Part model, mm, in its own coordinate system. Face numbers are marked on the shaded views. Give positions to 0.01 mm unless a question says otherwise; leave off trailing zeros. Write each loop counter-clockwise with the first axis right and the second up, starting at its lowest first coordinate (ties: lowest second). Pieces come first, ordered by that corner, then holes. Notation, with made-up numbers: M 54,44 L 65,44 A16 ccw 65,74 Z; hole C -20,-4 d2. An arc over 180 degrees is marked long. Use a Markdown table: item, result.
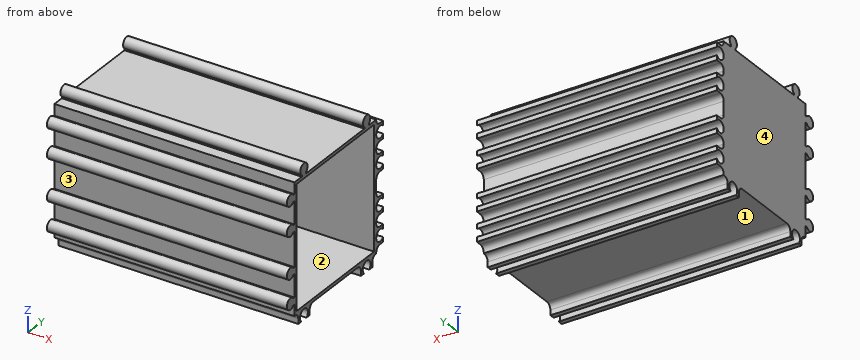
```python
from build123d import *

# Parameters (mm, degrees)
EXTRUDE_1_DEPTH             = 90
SKETCH_2_W                  = 90
SKETCH_2_H                  = 42.75
EXTRUDE_2_DEPTH             = 8.2
SKETCH_3_W                  = 90
SKETCH_3_H                  = 52.45
EXTRUDE_3_DEPTH             = 8.2
SKETCH_4_W                  = 3.95
SKETCH_4_H                  = 2.25
CUT_EXTRUDE_1_DEPTH         = 91
SKETCH_5_W                  = 3.95
SKETCH_5_H                  = 29.5
CUT_EXTRUDE_2_DEPTH         = 91
SKETCH_6_W                  = 3.95
SKETCH_6_H                  = 6.2
CUT_EXTRUDE_3_DEPTH         = 91
SKETCH_7_W                  = 2.25
SKETCH_7_H                  = 3.95
CUT_EXTRUDE_4_DEPTH         = 91
SKETCH_8_W                  = 4.5
SKETCH_8_H                  = 3.95
CUT_EXTRUDE_5_DEPTH         = 91
SKETCH_9_W                  = 9
SKETCH_9_H                  = 3.95
CUT_EXTRUDE_6_DEPTH         = 91
SKETCH_10_W                 = 4.5
SKETCH_10_H                 = 3.95
CUT_EXTRUDE_7_DEPTH         = 91
SKETCH_11_W                 = 2.25
SKETCH_11_H                 = 3.95
CUT_EXTRUDE_8_DEPTH         = 91
SKETCH_12_W                 = 46.1
SKETCH_12_H                 = 44.6
CUT_EXTRUDE_9_DEPTH         = 86.2
HOLE_WIZARD_2_5_2_5_1_D     = 2.5
HOLE_WIZARD_2_5_2_5_1_DEPTH = 90
HOLE_WIZARD_4_5_4_5_1_D     = 4.5
HOLE_WIZARD_4_5_4_5_1_DEPTH = 90
SKETCH_19_R                 = 1.67252853
SKETCH_19_R_2               = 1.459159852
SKETCH_19_R_3               = 1.459908976
SKETCH_19_R_4               = 1.592821911
SKETCH_19_R_5               = 1.532216665
SKETCH_19_R_6               = 1.596138091
EXTRUDE_4_DEPTH             = 90
FILLET_1_R                  = 2
FILLET_2_R                  = 2
FILLET_3_R                  = 2
FILLET_4_R                  = 2
FILLET_5_R                  = 2
FILLET_6_R                  = 2
FILLET_7_R                  = 2
FILLET_8_R                  = 2
FILLET_9_R                  = 2
FILLET_10_R                 = 2
FILLET_11_R                 = 2
FILLET_12_R                 = 2


with BuildPart() as part:
    # Эскиз1 → Бобышка-Вытянуть1 (new body)
    with BuildSketch(Plane(origin=(90, 0, 0), x_dir=(0, 0, -1), z_dir=(1, 0, 0))):
        with BuildLine():
            Line((6.75, 160.906238208), (6.75, 204.25))
            Line((6.75, 204.25), (-38.093761792, 204.25))
            ThreePointArc((-38.093761792, 204.25), (-41.825, 203), (-38.093761792, 201.75))
            Line((-38.093761792, 201.75), (-37.5, 201.75))
            Line((-37.5, 201.75), (-37.5, 168.25))
            Line((-37.5, 168.25), (-38.093761792, 168.25))
            ThreePointArc((-38.093761792, 168.25), (-41.825, 167), (-38.093761792, 165.75))
            Line((-38.093761792, 165.75), (-37.5, 165.75))
            Line((-37.5, 165.75), (-37.5, 161.5))
            Line((-37.5, 161.5), (-33.25, 161.5))
            Line((-33.25, 161.5), (-33.25, 160.906238208))
            ThreePointArc((-33.25, 160.906238208), (-32, 157.175), (-30.75, 160.906238208))
            Line((-30.75, 160.906238208), (-30.75, 161.5))
            Line((-30.75, 161.5), (-22.25, 161.5))
            Line((-22.25, 161.5), (-22.25, 160.906238208))
            ThreePointArc((-22.25, 160.906238208), (-21, 157.175), (-19.75, 160.906238208))
            Line((-19.75, 160.906238208), (-19.75, 161.5))
            Line((-19.75, 161.5), (-6.75, 161.5))
            Line((-6.75, 161.5), (-6.75, 160.906238208))
            ThreePointArc((-6.75, 160.906238208), (-5.5, 157.175), (-4.25, 160.906238208))
            Line((-4.25, 160.906238208), (-4.25, 161.5))
            Line((-4.25, 161.5), (4.25, 161.5))
            Line((4.25, 161.5), (4.25, 160.906238208))
            ThreePointArc((4.25, 160.906238208), (5.5, 157.175), (6.75, 160.906238208))
        make_face()
    extrude(amount=-EXTRUDE_1_DEPTH)

    # Эскиз2 → Бобышка-Вытянуть2 (add)
    with BuildSketch(Plane(origin=(0, 0, -6.75), x_dir=(-1, 0, 0), z_dir=(0, 0, -1))):
        with Locations((-45, 182.875)):
            Rectangle(SKETCH_2_W, SKETCH_2_H)
    extrude(amount=EXTRUDE_2_DEPTH)

    # Эскиз3 → Бобышка-Вытянуть3 (add)
    with BuildSketch(Plane(origin=(0, 204.25, 0), x_dir=(-1, 0, 0), z_dir=(0, 1, 0))):
        with Locations((-45, 11.275)):
            Rectangle(SKETCH_3_W, SKETCH_3_H)
    extrude(amount=EXTRUDE_3_DEPTH)

    # Эскиз4 → Вырез-Вытянуть1 (cut, through all)
    with BuildSketch(Plane.ZY):
        with Locations((-12.975, 162.625)):
            Rectangle(SKETCH_4_W, SKETCH_4_H)
    extrude(amount=-CUT_EXTRUDE_1_DEPTH, mode=Mode.SUBTRACT)

    # Эскиз5 → Вырез-Вытянуть2 (cut, through all)
    with BuildSketch(Plane.ZY):
        with Locations((-12.975, 185)):
            Rectangle(SKETCH_5_W, SKETCH_5_H)
    extrude(amount=-CUT_EXTRUDE_2_DEPTH, mode=Mode.SUBTRACT)

    # Эскиз6 → Вырез-Вытянуть3 (cut, through all)
    with BuildSketch(Plane.ZY):
        with Locations((-12.975, 209.35)):
            Rectangle(SKETCH_6_W, SKETCH_6_H)
    extrude(amount=-CUT_EXTRUDE_3_DEPTH, mode=Mode.SUBTRACT)

    # Эскиз7 → Вырез-Вытянуть4 (cut, through all)
    with BuildSketch(Plane.ZY):
        with Locations((-9.875, 210.475)):
            Rectangle(SKETCH_7_W, SKETCH_7_H)
    extrude(amount=-CUT_EXTRUDE_4_DEPTH, mode=Mode.SUBTRACT)

    # Эскиз8 → Вырез-Вытянуть5 (cut, through all)
    with BuildSketch(Plane.ZY):
        with Locations((0, 210.475)):
            Rectangle(SKETCH_8_W, SKETCH_8_H)
    extrude(amount=-CUT_EXTRUDE_5_DEPTH, mode=Mode.SUBTRACT)

    # Эскиз9 → Вырез-Вытянуть6 (cut, through all)
    with BuildSketch(Plane.ZY):
        with Locations((13.25, 210.475)):
            Rectangle(SKETCH_9_W, SKETCH_9_H)
    extrude(amount=-CUT_EXTRUDE_6_DEPTH, mode=Mode.SUBTRACT)

    # Эскиз10 → Вырез-Вытянуть7 (cut, through all)
    with BuildSketch(Plane.ZY):
        with Locations((26.5, 210.475)):
            Rectangle(SKETCH_10_W, SKETCH_10_H)
    extrude(amount=-CUT_EXTRUDE_7_DEPTH, mode=Mode.SUBTRACT)

    # Эскиз11 → Вырез-Вытянуть8 (cut, through all)
    with BuildSketch(Plane.ZY):
        with Locations((36.375, 210.475)):
            Rectangle(SKETCH_11_W, SKETCH_11_H)
    extrude(amount=-CUT_EXTRUDE_8_DEPTH, mode=Mode.SUBTRACT)

    # Эскиз12 → Вырез-Вытянуть9 (cut)
    with BuildSketch(Plane(origin=(90, 0, 0), x_dir=(0, 0, -1), z_dir=(1, 0, 0))):
        with Locations((-13.25, 185)):
            Rectangle(SKETCH_12_W, SKETCH_12_H)
    extrude(amount=-CUT_EXTRUDE_9_DEPTH, mode=Mode.SUBTRACT)

    # Диаметр отверстия Ø2.5 (2.5)1
    with Locations(Plane(origin=(90, 0, 0), x_dir=(0, 0, -1), z_dir=(1, 0, 0))):
        with Locations((5.5, 159.25), (-21, 159.25), (-5.5, 159.25), (-32, 159.25), (-39.75, 167), (-39.75, 203)):
            Hole(HOLE_WIZARD_2_5_2_5_1_D / 2, depth=HOLE_WIZARD_2_5_2_5_1_DEPTH)

    # Диаметр отверстия Ø4.5 (4.5)1
    with Locations(Plane.ZY):
        with Locations((-13.25, 167), (-13.25, 203), (-5.5, 210.75), (5.5, 210.75), (21, 210.75), (32, 210.75)):
            Hole(HOLE_WIZARD_4_5_4_5_1_D / 2, depth=HOLE_WIZARD_4_5_4_5_1_DEPTH)

    # Эскиз19 → Бобышка-Вытянуть4 (add)
    with BuildSketch(Plane(origin=(90, 0, 0), x_dir=(0, 0, -1), z_dir=(1, 0, 0))):
        with Locations((-39.75, 203)):
            Circle(SKETCH_19_R)
        with Locations((-39.75, 167)):
            Circle(SKETCH_19_R_2)
        with Locations((-32, 159.25)):
            Circle(SKETCH_19_R_3)
        with Locations((-21, 159.25)):
            Circle(SKETCH_19_R_4)
        with Locations((-5.5, 159.25)):
            Circle(SKETCH_19_R_5)
        with Locations((5.5, 159.25)):
            Circle(SKETCH_19_R_6)
    extrude(amount=-EXTRUDE_4_DEPTH)

    # Скругление1
    fillet_1_edges = [part.edges().sort_by_distance(p)[0] for p in [
        (45, 208.5, -8.75),
    ]]
    fillet(fillet_1_edges, radius=FILLET_1_R)

    # Скругление2
    fillet_2_edges = [part.edges().sort_by_distance(p)[0] for p in [
        (45, 163.75, -11),
    ]]
    fillet(fillet_2_edges, radius=FILLET_2_R)

    # Скругление3
    fillet_3_edges = [part.edges().sort_by_distance(p)[0] for p in [
        (45, 170.25, -11),
    ]]
    fillet(fillet_3_edges, radius=FILLET_3_R)

    # Скругление4
    fillet_4_edges = [part.edges().sort_by_distance(p)[0] for p in [
        (45, 199.75, -11),
    ]]
    fillet(fillet_4_edges, radius=FILLET_4_R)

    # Скругление5
    fillet_5_edges = [part.edges().sort_by_distance(p)[0] for p in [
        (45, 206.25, -11),
    ]]
    fillet(fillet_5_edges, radius=FILLET_5_R)

    # Скругление6
    fillet_6_edges = [part.edges().sort_by_distance(p)[0] for p in [
        (45, 208.5, -2.25),
    ]]
    fillet(fillet_6_edges, radius=FILLET_6_R)

    # Скругление7
    fillet_7_edges = [part.edges().sort_by_distance(p)[0] for p in [
        (45, 208.5, 2.25),
    ]]
    fillet(fillet_7_edges, radius=FILLET_7_R)

    # Скругление8
    fillet_8_edges = [part.edges().sort_by_distance(p)[0] for p in [
        (45, 208.5, 8.75),
    ]]
    fillet(fillet_8_edges, radius=FILLET_8_R)

    # Скругление9
    fillet_9_edges = [part.edges().sort_by_distance(p)[0] for p in [
        (45, 208.5, 17.75),
    ]]
    fillet(fillet_9_edges, radius=FILLET_9_R)

    # Скругление10
    fillet_10_edges = [part.edges().sort_by_distance(p)[0] for p in [
        (45, 208.5, 24.25),
    ]]
    fillet(fillet_10_edges, radius=FILLET_10_R)

    # Скругление11
    fillet_11_edges = [part.edges().sort_by_distance(p)[0] for p in [
        (45, 208.5, 28.75),
    ]]
    fillet(fillet_11_edges, radius=FILLET_11_R)

    # Скругление12
    fillet_12_edges = [part.edges().sort_by_distance(p)[0] for p in [
        (45, 208.5, 35.25),
    ]]
    fillet(fillet_12_edges, radius=FILLET_12_R)


solid = part.part
```
1. Cut at C-C, the plane z = 14. Give the cut face in (x, y).
Findings below:
| item | result |
|---|---|
| outline | M 0,161.5 L 90,161.5 L 90,162.7 L 3.8,162.7 L 3.8,207.3 L 90,207.3 L 90,208.5 L 0,208.5 Z |
2. Cut at D-D, the plane y = 174. Give the cut face in (x, z).
Findings below:
| item | result |
|---|---|
| outline | M 0,-11 L 90,-11 L 90,-9.8 L 3.8,-9.8 L 3.8,36.3 L 90,36.3 L 90,37.5 L 0,37.5 Z |
3. Cut at B-B, the plane y = 159.25. Give the cut face in (x, z) (3 decimals).
Findings below:
| item | result |
|---|---|
| outline | M 0,-7.575 L 90,-7.575 L 90,-3.425 L 0,-3.425 Z; M 0,3.425 L 90,3.425 L 90,7.575 L 0,7.575 Z; M 0,18.925 L 90,18.925 L 90,23.075 L 0,23.075 Z; M 0,29.925 L 90,29.925 L 90,34.075 L 0,34.075 Z |
4. Drop flat-ended pins along their axis: P1, Ø4, axis at x = 67, z = 13, coming from the +Y side; P2, Ø1.6, axis at x = 54, y = 211.5, coming from the +Z side; P3, Ø2, axis at x = 36.5, y = 211.5, coming from the -Z side; P4, Ø3.5, axis at y = 210.75, z = -5.5, coming from the -X side. Give the stop position or say it passes through.
Findings below:
| item | result |
|---|---|
| P1 | y = 208.5 |
| P2 | z = 35.25 |
| P3 | z = -8.75 |
| P4 | through |
5. Cut at A-A, the plane z = 39.75. Give the cut face in (x, y) (3 decimals), then the cut area to 3 significant figures.
Findings below:
| item | result |
|---|---|
| outline | M 0,164.925 L 90,164.925 L 90,169.075 L 0,169.075 Z; M 0,200.925 L 90,200.925 L 90,205.075 L 0,205.075 Z |
| area | 747 mm2 |
6. Drill centre lines: L1, parallel to Z at x = 61, y = 167 (3 decimals); L2, parallel to Z at x = 7, y = 184; L3, parallel to Y at x = 42.5, z = 34.5. Where is each one in solid material? Low to high.
Findings below:
| item | result |
|---|---|
| L1 | -11 to -9.8, 36.3 to 41.825 |
| L2 | -11 to -9.8, 36.3 to 37.5 |
| L3 | 161.5 to 162.7, 207.3 to 212.45 |
7. Two-plate mould, pull along Z, no slides. Class the marked faces 1, 2, 3 and 4: released by +Z, released by -Z, zero draft, split by the parting line, or undercut.
Findings below:
| item | result |
|---|---|
| face 1 | released by -Z |
| face 2 | undercut |
| face 3 | undercut |
| face 4 | zero draft |
